from build123d import *

# Parameters (mm, degrees)
BOSS_EXTRUDE1_DEPTH = 30
SKETCH2_W           = 61.936045122
SKETCH2_H           = 20
CUT_EXTRUDE1_DEPTH  = 92
SKETCH3_R           = 10
BOSS_EXTRUDE2_DEPTH = 40
SKETCH4_W           = 66.5
SKETCH4_H           = 18
BOSS_EXTRUDE3_DEPTH = 75
FILLET1_R           = 10
FILLET2_R           = 10


with BuildPart() as part:
    # Sketch1 → Boss-Extrude1 (new body)
    with BuildSketch(Plane.XY):
        with BuildLine():
            Line((-51.690581775, -18.31873005), (-37.309418225, -11.68126995))
            ThreePointArc((-37.309418225, -11.68126995), (-33.076645035, -7.99121144), (-31.5, -2.601676105))
            Line((-31.5, -2.601676105), (-31.5, 41))
            ThreePointArc((-31.5, 41), (-28.571067812, 48.071067812), (-21.5, 51))
            Line((-21.5, 51), (47.5, 51))
            ThreePointArc((47.5, 51), (54.571067812, 48.071067812), (57.5, 41))
            Line((57.5, 41), (57.5, 27))
            Line((57.5, 27), (47.5, 17))
            Line((47.5, 17), (28.5, 17))
            Line((28.5, 17), (28.5, 1))
            Line((28.5, 1), (18.5, -9))
            Line((18.5, -9), (13.5, -9))
            ThreePointArc((13.5, -9), (9.964466094, -10.464466094), (8.5, -14))
            Line((8.5, -14), (8.5, -51))
            Line((8.5, -51), (-47.5, -51))
            ThreePointArc((-47.5, -51), (-54.571067812, -48.071067812), (-57.5, -41))
            Line((-57.5, -41), (-57.5, -27.398323895))
            ThreePointArc((-57.5, -27.398323895), (-55.923354965, -22.00878856), (-51.690581775, -18.31873005))
        make_face()
    extrude(amount=BOSS_EXTRUDE1_DEPTH)

    # Sketch2 → Cut-Extrude1 (cut)
    with BuildSketch(Plane(origin=(0, 51, 0), x_dir=(1, 0, 0), z_dir=(0, 1, 0))):
        with Locations((-30.968022561, -15)):
            Rectangle(SKETCH2_W, SKETCH2_H)
    extrude(amount=-CUT_EXTRUDE1_DEPTH, mode=Mode.SUBTRACT)

    # Sketch3 → Boss-Extrude2 (add)
    with BuildSketch(Plane(origin=(0, 51, 0), x_dir=(1, 0, 0), z_dir=(0, 1, 0))):
        with Locations((28.75, -15)):
            Circle(SKETCH3_R)
    extrude(amount=BOSS_EXTRUDE2_DEPTH)

    # Sketch4 → Boss-Extrude3 (add)
    with BuildSketch(Plane(origin=(0, -41, 0), x_dir=(1, 0, 0), z_dir=(0, 1, 0))):
        with Locations((-34.25, -15)):
            Rectangle(SKETCH4_W, SKETCH4_H)
    extrude(amount=BOSS_EXTRUDE3_DEPTH)

    # Fillet1
    fillet1_edges = [part.edges().sort_by_distance(p)[0] for p in [
        (-67.5, -41, 15),
    ]]
    fillet(fillet1_edges, radius=FILLET1_R - 0.0001)  # a hair under: the kernel refuses the full size

    # Fillet2
    fillet2_edges = [part.edges().sort_by_distance(p)[0] for p in [
        (-67.5, 34, 15),
    ]]
    fillet(fillet2_edges, radius=FILLET2_R)


solid = part.part
Part model, mm, in its own coordinate system. A direction names the side the tool comes from. Give positions to 0.01 mm unless a question says otherwise; leave off trailing zeros. Write each loop counter-clockwise with the first axis right and the second up, starting at its lowest first coordinate (ties: lowest second). Pieces come first, ordered by that corner, then holes.
1) Two-plate mould, pull along Z, no slides. Class faces 5 (the face through (-28.65, 47.99, 27.46)), 6 (the face through (-30, 34, 15)), 7 (the face through (1, 1, 30)): released by +Z, released by -Z, zero draft, split by the parting line, or undercut.
Resolved:
face 5: zero draft
face 6: undercut
face 7: released by +Z
2) Which spindle directions (+Z, -Z, +X, -X, +Y, -Y) get a long thin tool onto all of the face, cutting with end or side? Do faces 1 (the face through (-33.12, -8.06, 2.46)), 2 (the face through (-55.97, -22.08, 27.46)), 3 (the face through (38, 17, 15)), 4 (the face through (38.29, 70.72, 12)). Say none if no direction does.
Resolved:
face 1: -Z, -X, +Y
face 2: +Z, -X, +Y
face 3: +Z, -Z, +X, -Y
face 4: +Y
3) Pin check, flat tips, straight feed: pin 1 (4 mm diameter, centred on x = 17, z = 20.5, fed in from -Y); pin 2 (2.5 mm diameter, centred on y = 28.5, z = 26.5, fed in from -X); pin 3 (3 mm diameter, centred on x = -2.5, z = 15.5, fed in from +Y). Stop position of each tip, or through.
Resolved:
pin 1: stops at y = -9
pin 2: stops at x = -31.5
pin 3: stops at y = 34
4) Probe L1, parallel to Z at x = -37.5, y = -35.5; L2, parallel to Y at x = -28.5, z = 20.75; L3, parallel to Y at x = 32.5, z = 8.25. List the from-to ranges inside material, lowest first.
Resolved:
L1: z = 0 to 5, 6 to 24, 25 to 30
L2: y = -51 to 34
L3: y = 17 to 91
5) Cut at C-C on x = 31.5. Write the cut outline in (y, z).
Resolved:
outline: (17, 0) - (51, 0) - (51, 5.39) - (91, 5.39) - (91, 24.61) - (51, 24.61) - (51, 30) - (17, 30) - close
6) Cut at D-D on y = 47.5. Write the cut outline in (x, z), then the cut area to 3 significant figures.
Resolved:
outline: (-29.1, 0) - (55.1, 0) - (55.1, 30) - (-29.1, 30) - (-29.1, 25) - (0, 25) - (0, 5) - (-29.1, 5) - close
area: 1,940 mm2
7) Cut at A-A on y = -29. Write the cut outline in (x, z), then the cut area to 3 significant figures.
Resolved:
outline: (-67.5, 6) - (-1, 6) - (-1, 24) - (-67.5, 24) - close; (-57.5, 0) - (8.5, 0) - (8.5, 30) - (-57.5, 30) - (-57.5, 25) - (0, 25) - (0, 5) - (-57.5, 5) - close
area: 2,030 mm2
8) Cut at B-B on z = 27. Write the cut outline in (x, y).
Resolved:
outline: (-57.5, -41) arc R10 ccw to (-47.5, -51) - (8.5, -51) - (8.5, -14) arc R5 cw to (13.5, -9) - (18.5, -9) - (28.5, 1) - (28.5, 17) - (47.5, 17) - (57.5, 27) - (57.5, 41) arc R10 ccw to (47.5, 51) - (-21.5, 51) arc R10 ccw to (-31.5, 41) - (-31.5, -2.6) arc R10 cw to (-37.31, -11.68) - (-51.69, -18.32) arc R10 ccw to (-57.5, -27.4) - close
